Check sheet for the drawn part. Datum: minimum x, y, z corner. Units: mm. A direction names the side the tool comes from. Coordinates: 2 decimals unless noted, no trailing zeros. Loops run counter-clockwise (first coordinate to the right, second up) from the corner with the lowest first, then second, coordinate; pieces in that order, holes last.
Q1. Sectioned sample at C-C (z = 22.5). Enter the section's corners in (x, y) (1 decimal).
Q2. Sectioned sample at A-A (x = 22.5). Enter the section's corners in (y, z) (1 decimal).
Q3. Sectioned sample at B-B (y = 2.75). Enter the section's corners in (x, z).
Q4. Mould release check, pull along Z, two halves, no side actions. Record for the marked faces 4, 5, 6 and 7: +Z half, -Z half, draft (parallel to the pull), parting line (faces both ways), or undercut.
Q5. Go/stop test with flat-tipped pins: P1, Ø4, axis at y = 10.5, z = 11.5, coming from the +X side; P2, Ø10, axis at x = 22, z = 18.5, coming from the -Y side (3 decimals); P3, Ø6, axis at x = 7.5, y = 4, coming from the -Z side. Record where each tip stops, or that it passes through.
Q6. Sectioned sample at D-D (x = 4). Enter the section's corners in (y, z) (1 decimal).
Q7. Access from +Z, -Z, +X, -X, +Y, -Y to the whole of each face (thin tool, end or side, straight path). Record for the marked faces 1, 2 and 3.
Q8. Material ranges on probe 1 along Z at (x, y) = (6.25, 8); probe 2 along X at (y, z) = (4.25, 13); probe 3 along Z at (x, y) = (17.5, 7.75), recorded low to high.
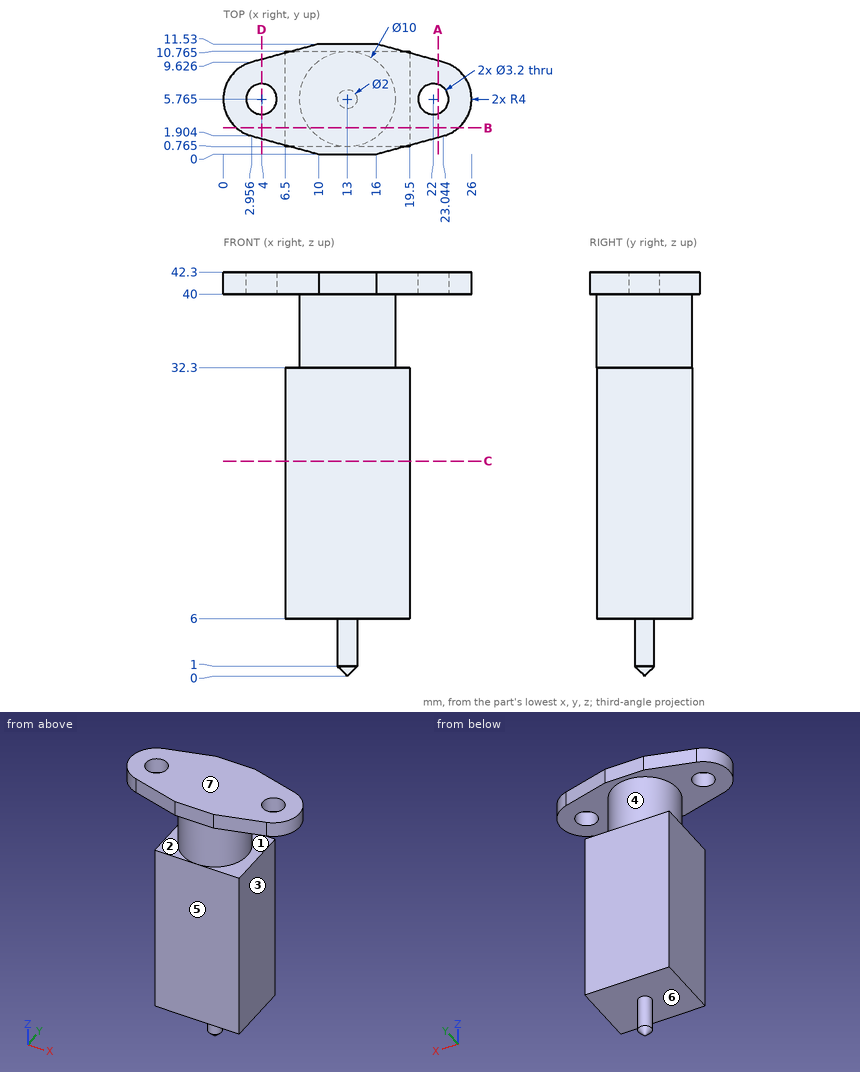
Geometry check:
1. outline: (6.5, 0.8) - (19.5, 0.8) - (19.5, 10.8) - (6.5, 10.8) - close
2. outline: (1.8, 40) - (4.2, 40) - (4.2, 42.3) - (1.8, 42.3) - close; (7.3, 40) - (9.8, 40) - (9.8, 42.3) - (7.3, 42.3) - close
3. outline: (1.37, 40) - (9.01, 40) - (9.01, 32.3) - (6.5, 32.3) - (6.5, 6) - (19.5, 6) - (19.5, 32.3) - (16.99, 32.3) - (16.99, 40) - (24.63, 40) - (24.63, 42.3) - (1.37, 42.3) - close
4. face 4: undercut
4. face 5: draft
4. face 6: -Z half
4. face 7: +Z half
5. P1: stops at x = 19.5
5. P2: stops at y = 0.765
5. P3: stops at z = 6
6. outline: (1.6, 40) - (4.2, 40) - (4.2, 42.3) - (1.6, 42.3) - close; (7.4, 40) - (9.9, 40) - (9.9, 42.3) - (7.4, 42.3) - close
7. face 1: +X
7. face 2: -X
7. face 3: -Z, +X, +Y, -Y
8. probe 1: z = 40 to 42.3
8. probe 2: x = 6.5 to 19.5
8. probe 3: z = 6 to 42.3
